```python
from build123d import *

# Parameters (mm, degrees)
F0_W     = 57.2733432055
F0_H     = 100.7320135832
F0_W_2   = 13.239064021
F0_H_2   = 0.7195146754
F1_DEPTH = 25.4
F2_R     = 3.0047813391
F2_R_2   = 2.9666314484
F3_DEPTH = 25.4


with BuildPart() as f1:
    # F0 (on Front) → F1 (new body)
    with BuildSketch(Plane.XZ):
        Polygon((-34.5366895199, 39.7171974182), (-31.3708260655, 35.9757170081), (25.9025171399, 35.9757170081), (25.9025171399, 39.7171974182), align=None)
        with Locations((-2.7341544628, -14.3902897835)):
            Rectangle(F0_W, F0_H)
        with Locations((9.2097852612, 26.6939844005)):
            Rectangle(F0_W_2, F0_H_2, mode=Mode.SUBTRACT)
        Polygon((-31.3708260655, -64.7562965751), (-31.3708260655, 35.9757170081), (-34.5366895199, 39.7171974182), (-34.5366895199, -65.907523036), align=None)
    extrude(amount=F1_DEPTH)

    # F2 (on face) → F3 (join)
    with BuildSketch(Plane.XZ.offset(25.4)):
        with Locations((-10.3610074148, 27.0537417382)):
            Circle(F2_R)
        with Locations((-2.7341544628, -60.4392103851)):
            Circle(F2_R_2)
    extrude(amount=F3_DEPTH)


solid = f1.part
```
Work out the finished part from the listing and answer in its coordinate system (mm). A direction names the side the tool comes from. Round coordinates to 2 decimals unless told otherwise and drop trailing zeros. Write each loop counter-clockwise with the first axis right and the second up, starting at its lowest first coordinate (ties: lowest second). Pieces come first, ordered by that corner, then holes.
1) Which of the six approach directions +Z, -Z, +X, -X, +Y, -Y give full straight-line access (tool end or side, diameter ignored) to faces 1 (the face through (-34.537, -13, -12)), 2 (the face through (-10.752, -37.922, 30.033))?
2) A cutting plane is placed at D-D on y = -46. Determine the outline of the cut face in (x, z), and give its area (3 significant figures).
3) A cutting plane is placed at B-B on z = -22.5. Determine the outline of the cut face in (x, y).
4) A cutting plane is placed at A-A on x = 5.5. Determine the outline of the cut face in (y, z).
5) Consider probe 1 along Y at (x, z) = (-31.5, -21.5); probe 2 along Z at (x, y) = (23, -7); probe 3 along X at (y, z) = (-35, 26). Determine where each line is inside the solid, lowest interval first.
6) A cutting plane is placed at C-C on x = -1.5. Determine the outline of the cut face in (y, z).
7) Flat-ended cylindrical pins translate along their axes: P1, Ø10.5, axis at x = 7, y = -13, coming from the -Z side; P2, Ø6, axis at x = -1.5, z = -33, coming from the -Y side; P3, Ø5, axis at x = 9.5, z = -14, coming from the +Y side; P4, Ø1, axis at x = -4.5, y = -31.5, coming from the -Z side. Find the tip coordinate at first contact, or state that the pin passes through.
8) Determine the mould class of faces 3 (the face through (9, -13, 26.334)), 4 (the face through (25.903, -13, -13)), 5 (the face through (-3, -13, -64.756)), 6 (the face through (9, -13, 27.054)) for opening direction X: pulls with the +X half, pulls with the -X half, needs draft (parallel to the pull), parting line crosses it, or undercut.
Entries:
1. face 1: +Z, -Z, -X, +Y, -Y
1. face 2: -Y
2. outline: circle Ø6.01 at (-10.36, 27.05); circle Ø5.93 at (-2.73, -60.44)
2. area: 56.0 mm2
3. outline: (-34.54, -25.4) - (25.9, -25.4) - (25.9, 0) - (-34.54, 0) - close
4. outline: (-25.4, -64.76) - (0, -64.76) - (0, 26.33) - (-25.4, 26.33) - close; (-25.4, 27.05) - (0, 27.05) - (0, 39.72) - (-25.4, 39.72) - close
5. probe 1: y = -25.4 to 0
5. probe 2: z = -64.76 to 39.72
5. probe 3: x = -13.17 to -7.55
6. outline: (-50.8, -63.14) - (-25.4, -63.14) - (-25.4, -64.76) - (0, -64.76) - (0, 39.72) - (-25.4, 39.72) - (-25.4, -57.74) - (-50.8, -57.74) - close
7. P1: stops at z = -64.76
7. P2: stops at y = -25.4
7. P3: stops at y = 0
7. P4: stops at z = -63.12
8. face 3: undercut
8. face 4: pulls with the +X half
8. face 5: needs draft
8. face 6: undercut
